Here's how the part is built. I have some questions about the finished solid (model axes, mm). A direction names the side the tool comes from. Coordinates: 2 decimals unless noted, no trailing zeros. Write each loop counter-clockwise with the first axis right and the second up, starting at its lowest first coordinate (ties: lowest second). Pieces come first, ordered by that corner, then holes. Notation, with made-up numbers: M -40,-12 L 13,-12 A15 cw 13,-8 Z; hole C -14.75,87.5 d3. An arc over 180 degrees is marked long. Use a Markdown table: item, result.
```python
from build123d import *

# Parameters (mm, degrees)
SKETCH_4_W               = 90
SKETCH_4_H               = 110
EXTRUDE_2_DEPTH          = 50
SHELL_2_T                = -1.5
SKETCH_5_W               = 4
SKETCH_5_H               = 4
CUT_EXTRUDE_2_DEPTH      = 50
MIRROR_5_COPY_1_SKETCH_W = 4
MIRROR_5_COPY_1_SKETCH_H = 4
MIRROR_5_COPY_1_DEPTH    = 50
SKETCH_9_R               = 20
CUT_EXTRUDE_5_DEPTH      = 50
SKETCH_12_W              = 23
SKETCH_12_H              = 23
CUT_EXTRUDE_6_DEPTH      = 50
SKETCH_15_R              = 1.25
CUT_EXTRUDE_8_DEPTH      = 129
SKETCH_16_W              = 27
SKETCH_16_H              = 20
CUT_EXTRUDE_9_DEPTH      = 50
SKETCH_17_R              = 1
CUT_EXTRUDE_10_DEPTH     = 50
SKETCH_19_R              = 1
CUT_EXTRUDE_11_DEPTH     = 50
SKETCH_21_R              = 1
CUT_EXTRUDE_12_DEPTH     = 50
SKETCH_22_R              = 1
CUT_EXTRUDE_13_DEPTH     = 50
FILLET_1_R               = 1
FILLET_2_R               = 1
SKETCH_25_W              = 40
SKETCH_25_H              = 5
CUT_EXTRUDE_15_DEPTH     = 50


with BuildPart() as part:
    # 草图4 → 凸台-拉伸2 (new body)
    with BuildSketch(Plane(origin=(0, 0, 0), x_dir=(1, 0, 0), z_dir=(0, 1, 0))):
        Rectangle(SKETCH_4_W, SKETCH_4_H)
    extrude(amount=EXTRUDE_2_DEPTH)

    # 抽壳2
    shell_2_openings = [part.faces().sort_by_distance(p)[0] for p in [
        (0, 50, 0),
    ]]
    offset(amount=SHELL_2_T, openings=shell_2_openings, kind=Kind.INTERSECTION)

    # 草图5 → 切除-拉伸2 (cut)
    with BuildSketch(Plane(origin=(0, 1.5, 0), x_dir=(1, 0, 0), z_dir=(0, 1, 0))):
        with Locations((-41.5, 51.5)):
            Rectangle(SKETCH_5_W, SKETCH_5_H)
    cut_extrude_2 = extrude(amount=-CUT_EXTRUDE_2_DEPTH, mode=Mode.SUBTRACT)

    # 镜向4: 切除-拉伸2 across plane
    add(cut_extrude_2.mirror(Plane.XY), mode=Mode.SUBTRACT)

    # 镜向5: 切除-拉伸2 across plane
    add(cut_extrude_2.mirror(Plane(origin=(0, 0, 0), x_dir=(0, 0, 1), z_dir=(1, 0, 0))), mode=Mode.SUBTRACT)

    # 镜向5 copy 1 sketch → 镜向5 copy 1 (cut)
    with BuildSketch(Plane(origin=(0, 1.5, 0), x_dir=(-1, 0, 0), z_dir=(0, 1, 0))):
        with Locations((-41.5, 51.5)):
            Rectangle(MIRROR_5_COPY_1_SKETCH_W, MIRROR_5_COPY_1_SKETCH_H)
    extrude(amount=-MIRROR_5_COPY_1_DEPTH, mode=Mode.SUBTRACT)

    # 草图9 → 切除-拉伸5 (cut)
    with BuildSketch(Plane(origin=(0, 1.5, 0), x_dir=(1, 0, 0), z_dir=(0, 1, 0))):
        Circle(SKETCH_9_R)
    extrude(amount=-CUT_EXTRUDE_5_DEPTH, mode=Mode.SUBTRACT)

    # 草图12 → 切除-拉伸6 (cut)
    with BuildSketch(Plane.XY.offset(55)):
        with Locations((-24.177084585, 23.410301274)):
            Rectangle(SKETCH_12_W, SKETCH_12_H)
    extrude(amount=-CUT_EXTRUDE_6_DEPTH, mode=Mode.SUBTRACT)

    # 草图15 → 切除-拉伸8 (cut)
    with BuildSketch(Plane.XY.offset(-53.5)):
        with Locations((-10.177084585, 23.410301274)):
            Circle(SKETCH_15_R)
        with Locations((-38.177084585, 23.410301274)):
            Circle(SKETCH_15_R)
    extrude(amount=CUT_EXTRUDE_8_DEPTH, mode=Mode.SUBTRACT)

    # 草图16 → 切除-拉伸9 (cut)
    with BuildSketch(Plane.XY.offset(55)):
        with Locations((22.5, 22)):
            Rectangle(SKETCH_16_W, SKETCH_16_H)
    extrude(amount=-CUT_EXTRUDE_9_DEPTH, mode=Mode.SUBTRACT)

    # 草图17 → 切除-拉伸10 (cut)
    with BuildSketch(Plane.XY.offset(55)):
        with Locations((35, 34)):
            Circle(SKETCH_17_R)
    extrude(amount=-CUT_EXTRUDE_10_DEPTH, mode=Mode.SUBTRACT)

    # 草图19 → 切除-拉伸11 (cut)
    with BuildSketch(Plane.XY.offset(55)):
        with Locations((35, 10)):
            Circle(SKETCH_19_R)
    extrude(amount=-CUT_EXTRUDE_11_DEPTH, mode=Mode.SUBTRACT)

    # 草图21 → 切除-拉伸12 (cut)
    with BuildSketch(Plane.XY.offset(55)):
        with Locations((10, 34)):
            Circle(SKETCH_21_R)
    extrude(amount=-CUT_EXTRUDE_12_DEPTH, mode=Mode.SUBTRACT)

    # 草图22 → 切除-拉伸13 (cut)
    with BuildSketch(Plane.XY.offset(55)):
        with Locations((10, 10)):
            Circle(SKETCH_22_R)
    extrude(amount=-CUT_EXTRUDE_13_DEPTH, mode=Mode.SUBTRACT)

    # 圆角1
    fillet_1_edges = [part.edges().sort_by_distance(p)[0] for p in [
        (-45, 25, -55),
        (45, 25, -55),
        (45, 25, 55),
        (-45, 25, 55),
    ]]
    fillet(fillet_1_edges, radius=FILLET_1_R)

    # 圆角2
    fillet_2_edges = [part.edges().sort_by_distance(p)[0] for p in [
        (0, 0, -55),
        (-45, 0, 0),
        (45, 0, 0),
        (0, 0, 55),
        (44.707106781, 0, 54.707106781),
        (-44.707106781, 0, 54.707106781),
        (-44.707106781, 0, -54.707106781),
        (44.707106781, 0, -54.707106781),
    ]]
    fillet(fillet_2_edges, radius=FILLET_2_R)

    # 草图25 → 切除-拉伸15 (cut)
    with BuildSketch(Plane(origin=(0, 0, 53.5), x_dir=(-1, 0, 0), z_dir=(0, 0, -1))):
        with Locations((-23.5, 47.5)):
            Rectangle(SKETCH_25_W, SKETCH_25_H)
    extrude(amount=-CUT_EXTRUDE_15_DEPTH, mode=Mode.SUBTRACT)


solid = part.part
```
1. Suppose I cut it at B-B on y = 18. Write out the boundary of the cut face in (x, z), and give its area (3 significant figures).
Answers follow:
| item | result |
|---|---|
| outline | M -45,-54 A1 ccw -44,-55 L 44,-55 A1 ccw 45,-54 L 45,54 A1 ccw 44,55 L 36,55 L 36,53.5 L 43.5,53.5 L 43.5,-53.5 L -43.5,-53.5 L -43.5,53.5 L -35.68,53.5 L -35.68,55 L -44,55 A1 ccw -45,54 Z; M -12.68,53.5 L 9,53.5 L 9,55 L -12.68,55 Z |
| area | 515 mm2 |
2. Which directions (+Z, -Z, +X, -X, +Y, -Y) give clear straight access to the entire face, cutting with the end or side of a thin tool? Please do faces 5 (the face through (-1, 25, -55)), 6 (the face through (-10.45, 22.19, 54.24)), 7 (the face through (-1, 25, -53.5)).
Answers follow:
| item | result |
|---|---|
| face 5 | -Z, +X, -X, +Y, -Y |
| face 6 | +Z |
| face 7 | +Y |
3. I need wall thicknesses on probe 1 along Z at (x, y) = (-2.5, 11.5); probe 2 along X at (y, z) = (21, 36); probe 3 along Y at (x, z) = (29, 29.5). Which ranges of each line are inside material? Lowest first, please.
Answers follow:
| item | result |
|---|---|
| probe 1 | z = -55 to -53.5, 53.5 to 55 |
| probe 2 | x = -45 to -43.5, 43.5 to 45 |
| probe 3 | y = 0 to 1.5 |
4. Suppose I cut it at C-C on z = 0. Write out the boundary of the cut face in (x, y).
Answers follow:
| item | result |
|---|---|
| outline | M -45,1 A1 ccw -44,0 L -20,0 L -20,1.5 L -43.5,1.5 L -43.5,50 L -45,50 Z; M 20,0 L 44,0 A1 ccw 45,1 L 45,50 L 43.5,50 L 43.5,1.5 L 20,1.5 Z |
5. Suppose I cut it at D-D on z = -32.5. Write out the boundary of the cut face in (x, y).
Answers follow:
| item | result |
|---|---|
| outline | M -45,1 A1 ccw -44,0 L 44,0 A1 ccw 45,1 L 45,50 L 43.5,50 L 43.5,1.5 L -43.5,1.5 L -43.5,50 L -45,50 Z |
6. Suppose I cut it at A-A on x = -23.5. Write out the boundary of the cut face in (y, z), and give its area (3 significant figures).
Answers follow:
| item | result |
|---|---|
| outline | M 0,-54 A1 ccw 1,-55 L 50,-55 L 50,-53.5 L 1.5,-53.5 L 1.5,53.5 L 11.91,53.5 L 11.91,55 L 1,55 A1 ccw 0,54 Z; M 34.91,53.5 L 50,53.5 L 50,55 L 34.91,55 Z |
| area | 276 mm2 |
7. We'd pull the mould along Y, two halves only. Please class faces 1 (the face through (-20.2, 0, -0.8)), 2 (the face through (-39.17, 22.65, 54.24)), 3 (the face through (-1, 25, 53.5)), 4 (the face through (-44, 50, 0)): +Y half, -Y half, draft (parallel to the pull), parting line (faces both ways), or undercut.
Answers follow:
| item | result |
|---|---|
| face 1 | -Y half |
| face 2 | undercut |
| face 3 | draft |
| face 4 | +Y half |
8. Will these pins go through, and if not, where does the flat tip stop? pin 1 Ø10 at (x, z) = (12, -15) entering from +Y; pin 2 Ø10 at (x, z) = (7, 25.5) entering from -Y; pin 3 Ø0.8 at (x, y) = (-42, 0.5) entering from -Z (3 decimals); pin 4 Ø1.6 at (x, z) = (25, 54.5) entering from +Y.
Answers follow:
| item | result |
|---|---|
| pin 1 | stops at y = 1.5 |
| pin 2 | stops at y = 0 |
| pin 3 | stops at z = -54.995 |
| pin 4 | stops at y = 45 |
